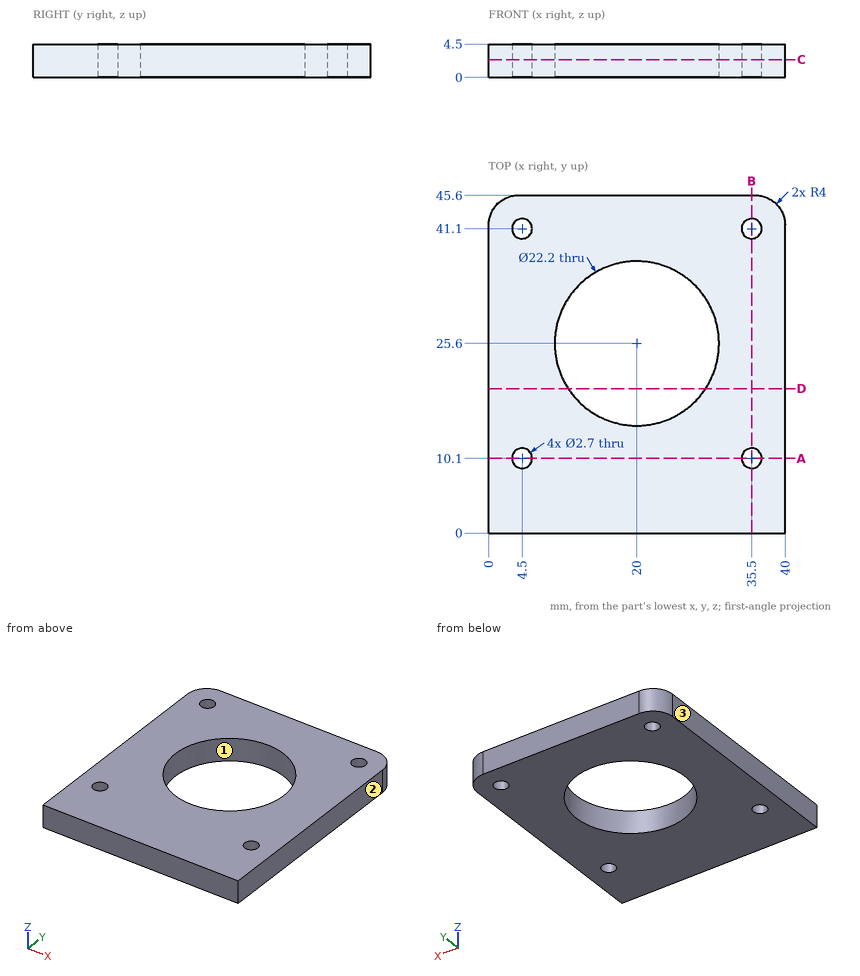
The drawing under review shows one solid part. Ordinate dimensions are in mm from its lowest x, y, z. Round coordinates to 2 decimals unless told otherwise and drop trailing zeros. Write each loop counter-clockwise with the first axis right and the second up, starting at its lowest first coordinate (ties: lowest second). Pieces come first, ordered by that corner, then holes. Notation, with made-up numbers: (20.25, -38) -> (75.25, -38) arc R33 cw to (75.25, -6) -> close; hole circle Ø8 at (51, 69.25). An arc over 180 degrees is marked (long way). One line per question, with ' | ' between items. Start each with the question number.
(1) For line 1 along Y through (x, z) = (35.5, 1.15); line 2 along Y through (x, z) = (36.5, 1.3); line 3 along Y through (x, z) = (13, 1.8), list the stretches that pass through material, from the lowest coordinate up. Write a range as from..to.
(2) Add section C-C, the plane z = 2.4. Write out the cut boundary in (x, y), plus the area to 3 significant figures.
(3) Insertion check: P1, Ø18, axis at x = 20, y = 25.6, coming from the +Z side. The pin has a flat end and moves straight along its axis. Give the tip position at first contact, or say it passes through.
(4) Add section D-D, the plane y = 19.5. Write out the cut boundary in (x, z).
(5) Mouldability with a two-part tool opening along X and no side actions: class the marked faces 1, 2 and 3 as released by +X, released by -X, zero draft, split by the parting line, or undercut.
(6) Add section A-A, the plane y = 10.1. Write out the cut boundary in (x, z), plus the area to 3 significant figures.
(7) Add section B-B, the plane x = 35.5. Write out the cut boundary in (y, z), plus the area to 3 significant figures.
Answer list:
1) line 1: 0..8.75, 11.45..39.75, 42.45..45.6 | line 2: 0..9.19, 11.01..40.19, 42.01..45.57 | line 3: 0..16.99, 34.21..45.6
2) outline: (0, 0) -> (40, 0) -> (40, 41.6) arc R4 ccw to (36, 45.6) -> (4, 45.6) arc R4 ccw to (0, 41.6) -> close; hole circle Ø2.7 at (4.5, 10.1); hole circle Ø2.7 at (4.5, 41.1); hole circle Ø22.2 at (20, 25.6); hole circle Ø2.7 at (35.5, 10.1); hole circle Ø2.7 at (35.5, 41.1) | area: 1,410 mm²
3) P1: through
4) outline: (0, 0) -> (10.73, 0) -> (10.73, 4.5) -> (0, 4.5) -> close; (29.27, 0) -> (40, 0) -> (40, 4.5) -> (29.27, 4.5) -> close
5) face 1: undercut | face 2: released by +X | face 3: released by -X
6) outline: (0, 0) -> (3.15, 0) -> (3.15, 4.5) -> (0, 4.5) -> close; (5.85, 0) -> (34.15, 0) -> (34.15, 4.5) -> (5.85, 4.5) -> close; (36.85, 0) -> (40, 0) -> (40, 4.5) -> (36.85, 4.5) -> close | area: 156 mm²
7) outline: (0, 0) -> (8.75, 0) -> (8.75, 4.5) -> (0, 4.5) -> close; (11.45, 0) -> (39.75, 0) -> (39.75, 4.5) -> (11.45, 4.5) -> close; (42.45, 0) -> (45.6, 0) -> (45.6, 4.5) -> (42.45, 4.5) -> close | area: 181 mm²
